from build123d import *

# Parameters (mm, degrees)
F0_R          = 9.1821
F1_DEPTH      = 15.24
F3_DEPTH      = 9.1831
F3_DEPTH_BACK = 9.1831


with BuildPart() as f1:
    # F0 (on Top) → F1 (new body)
    with BuildSketch(Plane.XY):
        Circle(F0_R)
    extrude(amount=-F1_DEPTH)

    # F2 (on Front) → F3 (cut, two sides)
    with BuildSketch(Plane.XZ) as f3_sk:
        Polygon((-9.1821, 0), (-9.1821, -12.7), (-6.6421, -12.7), (-5.3721, -12.7), (-5.3721, -10.16), (-6.6421, -10.16), (-6.6421, 0), align=None)
        Polygon((9.1821, -12.7), (9.1821, 0), (6.6421, 0), (6.6421, -10.16), (5.3721, -10.16), (5.3721, -12.7), (6.6421, -12.7), align=None)
    extrude(amount=-F3_DEPTH, mode=Mode.SUBTRACT)
    extrude(f3_sk.sketch, amount=F3_DEPTH_BACK, mode=Mode.SUBTRACT)

    # F4 (on Front) → F5 (revolve)
    with BuildSketch(Plane.XZ):
        Polygon((0, 32.639), (0, 0), (3.175, 0), (3.175, 28.1854718924), align=None)
    revolve(axis=Axis((0, 0, 15.3003977612), (0, 0, 1)))


solid = f1.part
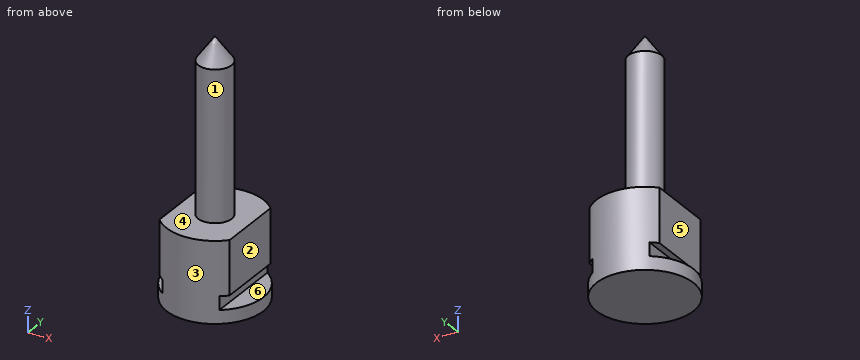
Model file for the job. Use its own axes, mm. Face numbers are marked on the shaded views. A direction names the side the tool comes from. Round coordinates to 2 decimals unless told otherwise and drop trailing zeros. Order: outer loops, then holes, each group sorted by start corner. A loop starts at its lowest first (then second) coordinate and runs counter-clockwise, first axis right, second up.
(1) Pull direction Z, two halves, no side cores. Call the marked faces 4, 5 and 6: released by +Z, released by -Z, zero draft, split by the parting line, or undercut.
(2) Band-saw the part on A-A (y = 7). List the corners of the cut face in (x, z), then the cut area to 3 significant figures.
(3) Pin check, flat tips, straight feed: pin 1 (4 mm diameter, centred on x = -2.5, y = 1.5, fed in from +Z); pin 2 (4 mm diameter, centred on x = 6.5, y = -3.5, fed in from +Z); pin 3 (10 mm diameter, centred on x = -1.5, z = -9, fed in from +Y); pin 4 (10 mm diameter, centred on y = 3, z = 28, fed in from -X) (3 decimals). Stop position of each tip, or through.
(4) Band-saw the part on B-B (z = 5). List the corners of the cut face in (x, y) (3 decimals).
(5) Band-saw the part on C-C (x = 4). List the corners of the cut face in (y, z), then the cut area to 3 significant figures.
(6) Band-saw the part on D-D (z = -6). List the corners of the cut face in (x, y), then the cut area to 3 significant figures.
(7) 3-axis set-ups, long thin cutter, end or side, ignore diameter. For the marked faces 1, 2 and 3: which of +Z, -Z, +X, -X, +Y, -Y reach the whole face in a straight line?
(8) Drill centre lines: line 1 (Z direction, x = 5.75, y = 2.5); line 2 (Z direction, x = -3.5, y = -3.75); line 3 (X direction, y = 3.5, z = -10). Where is each one in solid material? Low to high.
Verdict:
1. face 4: released by +Z
1. face 5: zero draft
1. face 6: undercut
2. outline: (-5.94, -15.24) - (5.94, -15.24) - (5.94, -12.7) - (5.37, -12.7) - (5.37, -10.16) - (5.94, -10.16) - (5.94, 0) - (-5.94, 0) - (-5.94, -10.16) - (-5.37, -10.16) - (-5.37, -12.7) - (-5.94, -12.7) - close
2. area: 178 mm2
3. pin 1: stops at z = 31.35
3. pin 2: stops at z = 0
3. pin 3: stops at y = 9.18
3. pin 4: stops at x = -3.175
4. outline: circle Ø6.35 at (0, 0)
5. outline: (-8.27, -15.24) - (8.27, -15.24) - (8.27, 0) - (-8.27, 0) - close
5. area: 252 mm2
6. outline: (-6.64, -6.34) arc R9.18 ccw to (6.64, -6.34) - (6.64, 6.34) arc R9.18 ccw to (-6.64, 6.34) - close
6. area: 221 mm2
7. face 1: +Z
7. face 2: +Z, +X, +Y, -Y
7. face 3: +Z, -Z
8. line 1: z = -15.24 to -12.7, -10.16 to 0
8. line 2: z = -15.24 to 0
8. line 3: x = -6.64 to 6.64
